from build123d import *

# Parameters (mm, degrees)
F0_W     = 110
F0_H     = 65
F1_DEPTH = 5
F2_R     = 3.1
F3_DEPTH = 25


with BuildPart() as f1:
    # F0 (on Right) → F1 (new body)
    with BuildSketch(Plane.YZ):
        Rectangle(F0_W, F0_H)
    extrude(amount=F1_DEPTH)

    # F2 (on face) → F3 (cut)
    with BuildSketch(Plane.YZ.offset(5)):
        with Locations((0, 12.6)):
            Circle(F2_R)
    extrude(amount=-F3_DEPTH, mode=Mode.SUBTRACT)


solid = f1.part
Read the model definition and answer for the solid it produces. Units are mm, in the model's axes. Round coordinates to 2 decimals unless told otherwise and drop trailing zeros. Loops run counter-clockwise (first coordinate to the right, second up) from the corner with the lowest first, then second, coordinate; pieces in that order, holes last.
Q1. Section A-A on z = 12.6 is taken. Write down the section's boundary in (x, y).
Q2. Determine the mould class of faces 1 (the face through (2, -1, -32.5)), 2 (the face through (5, -1, 0)), 3 (the face through (2.535, -0.672, 9.574)), 4 (the face through (2, -1, 32.5)) for opening direction Z: released by +Z, released by -Z, zero draft, split by the parting line, or undercut.
Q3. Consider probe 1 along Z at (x, y) = (3.25, 0). Determine where the line is inside the solid, lowest interval first.
Q4. Section B-B on y = 0 is taken. Write down the section's boundary in (x, z).
Output:
1. outline: (0, -55) - (5, -55) - (5, -3.1) - (0, -3.1) - close; (0, 3.1) - (5, 3.1) - (5, 55) - (0, 55) - close
2. face 1: released by -Z
2. face 2: zero draft
2. face 3: undercut
2. face 4: released by +Z
3. probe 1: z = -32.5 to 9.5, 15.7 to 32.5
4. outline: (0, -32.5) - (5, -32.5) - (5, 9.5) - (0, 9.5) - close; (0, 15.7) - (5, 15.7) - (5, 32.5) - (0, 32.5) - close
